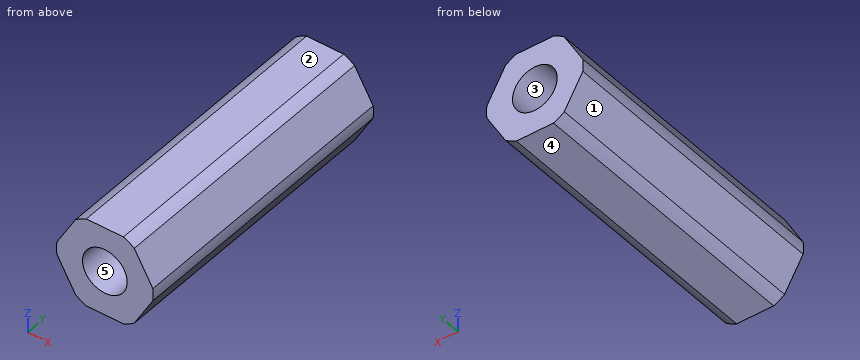
Autodesk Inventor part; units mm, degrees
ref_plane "YZ Plane" through (0, 0, 0) normal (1, 0, 0) x (0, 1, 0)
ref_plane "XZ Plane" through (0, 0, 0) normal (0, 1, 0) x (-1, 0, 0)
ref_plane "XY Plane" through (0, 0, 0) normal (0, 0, 1) x (1, 0, 0)
sketch "Sketch1" plane through (0, 0, 0) normal (0, 1, 0) x (-1, 0, 0)
  line L0 (-7.3323, 0) -> (-3.6662, 6.35)
  line L1 (-3.6662, 6.35) -> (3.6662, 6.35)
  line L2 (3.6662, 6.35) -> (7.3323, 0)
  line L3 (7.3323, 0) -> (3.6662, -6.35)
  line L4 (3.6662, -6.35) -> (-3.6662, -6.35)
  line L5 (-3.6662, -6.35) -> (-7.3323, 0)
  circle A0 centre (0, 0) radius 6.875
  circle A1 centre (0, 0) radius 6.35
  line L6 (-2.7496, -4.7625) -> (2.7496, -4.7625)
  line L7 (2.7496, -4.7625) -> (5.4993, 0)
  line L8 (5.4993, 0) -> (2.7496, 4.7625)
  line L9 (2.7496, 4.7625) -> (-2.7496, 4.7625)
  line L10 (-2.7496, 4.7625) -> (-5.4993, 0)
  line L11 (-5.4993, 0) -> (-2.7496, -4.7625)
  circle A2 centre (0, 0) radius 4.7625
  circle A3 centre (0, 0) radius 5.125
  circle A4 centre (0, 0) radius 9.525
  circle A5 centre (0, 0) radius 5.9436
  circle A6 centre (0, 0) radius 2.5527
  circle A7 centre (0, 0) radius 2.0193
  circle A8 centre (0, 0) radius 3.175
  circle A9 centre (0, 0) radius 8.7313
  point P0 (-4.1818, 5.457)
  point P1 (-2.635, 6.35)
  point P2 (-6.8168, -0.893)
  point P3 (-6.8168, 0.893)
  point P4 (-2.635, -6.35)
  point P5 (-4.1818, -5.457)
  point P6 (4.1818, -5.457)
  point P7 (2.635, -6.35)
  point P8 (6.8168, -0.893)
  point P9 (6.8168, 0.893)
  point P10 (2.635, 6.35)
  point P11 (4.1818, 5.457)
  point P12 (3.1778, -4.0208)
  point P13 (1.8932, -4.7625)
  point P14 (5.071, -0.7417)
  point P15 (5.071, 0.7417)
  point P16 (1.8932, 4.7625)
  point P17 (3.1778, 4.0208)
  point P18 (-3.1778, 4.0208)
  point P19 (-1.8932, 4.7625)
  point P20 (-5.071, -0.7417)
  point P21 (-5.071, 0.7417)
  point P22 (-1.8932, -4.7625)
  point P23 (-3.1778, -4.0208)
  dimension "d0" = 12.7
  dimension "d1" = 13.75
  dimension "d2" = 12.7
  dimension "d3" = 9.525
  dimension "d4" = 10.25
  dimension "d5" = 19.05
  dimension "d6" = 11.8872
  dimension "d7" = 5.1054
  dimension "d8" = 4.0386
  dimension "d9" = 6.35
  dimension "d153" = 0.7937
extrude "BaseProfile625Round" add sketch "Sketch1" along normal mid plane 40.894 contours L0 A0 L5 | A0 L0 | L0 A1 L5 A0 | L5 A0 | L0 A0 L1 A1 | A1 | L0 L1 A0 | A1 L4 A0 L5 | A0 L4 L5 | L1 A0 | L1 A0 L2 A1 | A1 L3 A0 L4 | L4 A0 | L1 L2 A0 | L2 A0 | L2 A0 L3 A1 | A0 L3 L4 | L3 A0 | L2 L3 A0 | L11 A3 L6 | A3 L11 A2 L6 | L6 A3 | A3 L11 | A2 L7 A3 L6 | A2 | A3 L7 L6 | L11 A3 L10 A2 | L11 L10 A3 | L7 A3 | A2 L8 A3 L7 | L10 A3 | L10 A3 L9 A2 | A3 L8 L7 | L10 L9 A3 | L9 A3 | L9 A3 L8 A2 | L8 A3 | L9 L8 A3 | A4 | A5 | A6 | A7 | A8 | A9
extrude "BaseProfileRoundTube" [suppressed]
extrude "BaseProfile500Hex" [suppressed]
extrude "BaseProfile500Thunderhex" cut sketch "Sketch1" along normal mid plane 914.4 contours L0 A0 L5 | A0 L0 | L5 A0 | L0 L1 A0 | A0 L4 L5 | L1 A0 | L4 A0 | L1 L2 A0 | L2 A0 | A0 L3 L4 | L3 A0 | L2 L3 A0 | A4 | A9
extrude "BaseProfile500Round" [suppressed]
extrude "BaseProfile375Hex" [suppressed]
extrude "BaseProfile375Thunderhex" [suppressed]
extrude "BaseProfile375Round" [suppressed]
extrude "TopShaftProfile1Hex500" [suppressed]
extrude "TopShaftProfile1ThunderHex500" [suppressed]
extrude "TopShaftProfile1Round500" [suppressed]
extrude "TopShaftProfile1Hex375" [suppressed]
extrude "TopShaftProfile1ThunderHex375" [suppressed]
extrude "TopShaftProfile1Round375" [suppressed]
extrude "TopShaftProfile2ThunderHex500" [suppressed]
extrude "TopShaftProfile2Round500" [suppressed]
extrude "TopShaftProfile2Hex375" [suppressed]
extrude "TopShaftProfile2ThunderHex375" [suppressed]
extrude "TopShaftProfile2Round375" [suppressed]
sketch "Sketch2" plane through (0, 0, 0) normal (1, 0, 0) x (0, 1, 0)
  line L0 (-40.8112, 0) -> (47.9537, 0)
  line L1 (0, -2.6658) -> (0, 15.9951)
  line L2 (27.5895, 4.4704) -> (28.7325, 4.4704)
  line L3 (28.7325, 4.4704) -> (28.7325, 4.7625)
  line L4 (28.7325, 4.7625) -> (29.812, 4.7625)
  line L5 (29.812, 4.7625) -> (30.32, 4.2545)
  line L6 (30.32, 4.2545) -> (30.32, 0)
  line L7 (27.5895, 4.4704) -> (27.5895, 0) construction
  line L8 (27.5895, 4.4704) -> (27.5895, 4.7625)
  line L9 (27.5895, 4.7625) -> (20.447, 4.7625)
  line L10 (20.447, 4.7625) -> (20.447, 0)
  line L11 (20.447, 0) -> (30.32, 0)
  line L12 (-20.447, 5.9436) -> (-21.59, 5.9436)
  line L13 (-21.59, 5.9436) -> (-21.59, 6.35)
  line L14 (-21.59, 6.35) -> (-22.6695, 6.35)
  line L15 (-22.6695, 6.35) -> (-23.1775, 5.842)
  line L16 (-23.1775, 5.842) -> (-23.1775, 0)
  line L17 (-20.447, 5.9436) -> (-20.447, 0) construction
  line L18 (-20.447, 5.9436) -> (-20.447, 6.35)
  line L19 (-20.447, 6.35) -> (-20.447, 6.35)
  line L20 (-20.447, 6.35) -> (-20.447, 0)
  line L21 (-20.447, 0) -> (-23.1775, 0)
  line L22 (0, 0) -> (0, 13.3292)
  line L23 (20.447, 0) -> (20.447, 4.7625)
  point P0 (25.4, 5.9436)
  point P1 (-23.1775, 0)
  point P2 (-20.447, 0)
  point P3 (30.955, 4.7625)
  point P4 (-17.4625, 6.2865)
  point P5 (25.4, 4.7625)
  point P6 (19.4005, 4.7625)
  point P7 (-25.4, 4.7625)
  point P8 (-26.543, 4.7625)
  dimension "TopBearingRoundDia2" = 9.525
  dimension "d65" = 45
  dimension "RetainingRingChamferSize2" = 0.508
  dimension "d72" = 20.447
  dimension "TopSnapRingDia2" = 8.9408
  dimension "d119" = 0.508
  dimension "d120" = 45
  dimension "d135" = 20.447
  dimension "d138" = 30.32
  dimension "d139" = 28.7325
  dimension "d140" = 27.5895
  dimension "d141" = 11.8872
  dimension "d142" = 12.7
  dimension "d143" = 21.59
  dimension "d144" = 20.447
  dimension "d145" = 23.1775
revolve "TopRetentionGroove&BearingRound" [suppressed]
sketch "Sketch3" plane through (0, 20.447, 0) normal (0, 1, 0) x (1, 0, 0)
  point P0 (0, 0)
  point P1 (0, 0)
hole "TopShaftTappedHole" at (0, 20.447, 0) direction (0, -1, 0) diameter 6.35 depth 15.875 tip angle 118
thread "TopShaftThread"
extrude "BottomShaftProfile1Hex500" [suppressed]
extrude "BottomShaftProfile1ThunderHex500" [suppressed]
extrude "BottomShaftProfile1Round500" [suppressed]
extrude "BottomShaftProfile1Hex375" [suppressed]
extrude "BottomShaftProfile1ThunderHex375" [suppressed]
extrude "BottomShaftProfile2ThunderHex500" [suppressed]
extrude "BottomShaftProfile1Round375" [suppressed]
extrude "BottomShaftProfile2Round500" [suppressed]
extrude "BottomShaftProfile2Hex375" [suppressed]
extrude "BottomShaftProfile2ThunderHex375" [suppressed]
extrude "BottomShaftProfile2Round375" [suppressed]
sketch "Sketch4" plane through (0, -20.447, 0) normal (0, -1, 0) x (1, 0, 0)
  point P0 (0, 0)
  point P1 (0, 0)
hole "BottomShaftTappedHole" at (0, -20.447, 0) direction (0, 1, 0) diameter 6.35 depth 15.875 tip angle 118
thread "BottomShaftThread"
revolve "BottomRetentionGroove&BearingRound" [suppressed]
extrude "BaseProfile375ThunderhexHole" [suppressed]
extrude "BaseProfile500ThunderhexHole" cut sketch "Sketch1" along normal mid plane 914.4 contours A6 | A7
equation "\"d18\" = BottomShaftProfile1Depth + TopShaftProfile1Depth + BaseShaftLength + TopShaftProfile2Depth + BottomShaftProfile2Depth"
equation "\"d72\" = 0.5 * d18"
equation "\"BaseShaftLength\" = 40.894"
equation "\"TopShaftProfile1Depth\" = 0"
equation "\"TopShaftProfile2Depth\" = 0"
equation "\"BottomShaftProfile1Depth\" = 0"
equation "\"BottomShaftProfile2Depth\" = 0"
equation "\"TopShaftHoleDia\" = 6.35"
equation "\"BottomShaftHoleDia\" = 6.35"
equation "\"TopBearingRoundDia\" = 9.525"
equation "\"TopGrooveWidth\" = 1.143"
equation "\"TopBearingRoundDistance\" = 7.14248"
equation "\"TopSnapRingDia\" = 8.9408"
equation "\"BottomBearingRoundDia\" = 12.7"
equation "\"BottomGrooveWidth\" = 1.143"
equation "\"BottomBearingRoundDistance\" = 0"
equation "\"BottomSnapRingDia\" = 11.8872"
equation "\"RoundTubeDia\" = 19.05"
properties part number "GreyT Claw 2 Gearbox Shaft" material "Aluminum 6061"
Design review of the part built by this model. Coordinates are the model's own, in mm. Face numbers are marked on the shaded views. A direction names the side the tool comes from. Coordinates: 2 decimals unless noted, no trailing zeros. Loops run counter-clockwise (first coordinate to the right, second up) from the corner with the lowest first, then second, coordinate; pieces in that order, holes last.
Item 1: Add section D-D (y = -1). Write out the cut boundary in (x, z) (3 decimals).
Completed:
outline: (-6.817, -0.893) - (-4.182, -5.457) arc R6.875 ccw to (-2.635, -6.35) - (2.635, -6.35) arc R6.875 ccw to (4.182, -5.457) - (6.817, -0.893) arc R6.875 ccw to (6.817, 0.893) - (4.182, 5.457) arc R6.875 ccw to (2.635, 6.35) - (-2.635, 6.35) arc R6.875 ccw to (-4.182, 5.457) - (-6.817, 0.893) arc R6.875 ccw to start; hole circle Ø5.105 at (0, 0)
Item 2: Add section C-C (y = -7.5). Write out the cut boundary in (x, z) (3 decimals), and give its area (3 significant figures).
Completed:
outline: (-6.817, -0.893) - (-4.182, -5.457) arc R6.875 ccw to (-2.635, -6.35) - (2.635, -6.35) arc R6.875 ccw to (4.182, -5.457) - (6.817, -0.893) arc R6.875 ccw to (6.817, 0.893) - (4.182, 5.457) arc R6.875 ccw to (2.635, 6.35) - (-2.635, 6.35) arc R6.875 ccw to (-4.182, 5.457) - (-6.817, 0.893) arc R6.875 ccw to start; hole circle Ø6.35 at (0, 0)
area: 106 mm2
Item 3: Add section A-A (x = 0). Write out the cut boundary in (y, z) (3 decimals), and give its area (3 significant figures).
Completed:
outline: (-20.447, -6.35) - (20.447, -6.35) - (20.447, -3.175) - (4.572, -3.175) - (4.198, -2.553) - (-4.198, -2.553) - (-4.572, -3.175) - (-20.447, -3.175) - close; (-20.447, 3.175) - (-4.572, 3.175) - (-4.198, 2.553) - (4.198, 2.553) - (4.572, 3.175) - (20.447, 3.175) - (20.447, 6.35) - (-20.447, 6.35) - close
area: 271 mm2
Item 4: For the marked faces 4 and 5, list the 3-axis set-ups (+Z, -Z, +X, -X, +Y, -Y) from which the entire face can be reached by the end or side of a thin tool; tool diameter is ignored.
Completed:
face 4: -Z, +X, -X, +Y, -Y
face 5: -Y
Item 5: Draft analysis for pull direction X (two halves, no side actions). For the marked faces 1, 2 and 3, state which applies: pulls with the +X half, pulls with the -X half, needs draft (parallel to the pull), parting line crosses it, or undercut.
Completed:
face 1: pulls with the -X half
face 2: needs draft
face 3: undercut
Item 6: Add section B-B (z = 0). Write out the cut boundary in (x, y) (3 decimals), and give its area (3 significant figures).
Completed:
outline: (-6.875, -20.447) - (-3.175, -20.447) - (-3.175, -4.572) - (-2.553, -4.198) - (-2.553, 4.198) - (-3.175, 4.572) - (-3.175, 20.447) - (-6.875, 20.447) - close; (2.553, -4.198) - (3.175, -4.572) - (3.175, -20.447) - (6.875, -20.447) - (6.875, 20.447) - (3.175, 20.447) - (3.175, 4.572) - (2.553, 4.198) - close
area: 314 mm2
Item 7: Wall thickness on L1, parallel to Z at x = 0, y = -10 (3 decimals); L2, parallel to X at y = -10, z = 0 (3 decimals); L3, parallel to X at y = -1, z = 0 (3 decimals): over which ranges is each line inside the solid? List them lowest first.
Completed:
L1: z = -6.35 to -3.175, 3.175 to 6.35
L2: x = -6.875 to -3.175, 3.175 to 6.875
L3: x = -6.875 to -2.553, 2.553 to 6.875
Item 8: Clearance check with flat-ended pins moving along their axes: pin 1 (3 mm diameter, centred on y = 15, z = -4.5, fed in from +X); pin 2 (5.5 mm diameter, centred on x = 0, z = 0, fed in from +Y); pin 3 (4 mm diameter, centred on x = 5, y = -11.5, fed in from -Z). State where each tip first meets the part, or that it passes through.
Completed:
pin 1: stops at x = 5.6
pin 2: stops at y = 4.32
pin 3: stops at z = -6.19
